```python
from build123d import *

# Parameters (mm, degrees)
F1_DEPTH = 161
F3_DEPTH = 161
F5_DEPTH = 161


with BuildPart() as f1:
    # F0 (on Top) → F1 (new body)
    with BuildSketch(Plane.XY):
        Polygon((800, 0), (0, 0), (0, -250), (28.50642, -318.820585), (81.179415, -371.49358), (150, -400), (800, -400), align=None)
    extrude(amount=-F1_DEPTH)

    # F2 (on face) → F3 (join)
    with BuildSketch(Plane(origin=(0, 0, -161), x_dir=(1, 0, 0), z_dir=(0, 0, -1))):
        Polygon((-191.910937, 466.098754), (-260, 301.717216), (-260, 0), (800, 0), (800, 660), (98.282784, 660), (-66.098754, 591.910937), align=None)
    extrude(amount=F3_DEPTH)

    # F4 (on face) → F5 (join)
    with BuildSketch(Plane(origin=(0, 0, -322), x_dir=(1, 0, 0), z_dir=(0, 0, -1))):
        Polygon((-412.328294, 613.376924), (-520, 353.434431), (-520, 0), (800, 0), (800, 920), (46.565569, 920), (-213.376924, 812.328294), align=None)
    extrude(amount=F5_DEPTH)


solid = f1.part
```
The model under review builds one solid part; all positions refer to its coordinate system, in mm. A direction names the side the tool comes from. Coordinates: 2 decimals unless noted, no trailing zeros. Order: outer loops, then holes, each group sorted by start corner. A loop starts at its lowest first (then second) coordinate and runs counter-clockwise, first axis right, second up. Notation, with made-up numbers: (42.5, 0.5) -> (91.5, 0.5) arc R23 cw to (91.5, 15.5) -> close; hole circle Ø2 at (84.25, -39.5). An arc over 180 degrees is marked (long way). Answer in a Markdown table with one row per item. Add a question column.
Item 1: We need section B-B on x = 546. Write out the cut boundary in (y, z).
Item 2: We need section C-C on z = -410. Write out the cut boundary in (x, y), plus the area to 3 significant figures.
Item 3: We need section D-D on z = -296. Write out the cut boundary in (x, y).
Item 4: We need section A-A on y = -159. Write out the cut boundary in (x, z).
Item 5: To check wall thickness, follow probe 1 along Z at (x, y) = (-190, -515); probe 2 along Z at (x, y) = (637, -542); probe 3 along X at (y, z) = (-105, -279). State the ranges of each line that lie inside material, in increasing order.
Item 6: Machinability: for faces 1 (the flat face through (454, -660, -240)), 2 (the flat face through (115.11, -385.55, -79.37)), 3 (the flat face through (-81.586, -866.918, -401.373)), 4 (the flat face through (-260, -153, -240)), which of the approach directions +Z, -Z, +X, -X, +Y, -Y give a long, thin tool a straight path to every point of the face, cutting with its end or side? Answer none if there is none.
Item 7: Clearance check with flat-ended pins moving along their axes: pin 1 (2 mm diameter, centred on x = 505.5, y = -748.5, fed in from +Z); pin 2 (2 mm diameter, centred on y = -513.5, z = -306, fed in from -X). State where each tip first meets the part, or that it passes through.
Final values:
| question | item | result |
|---|---|---|
| 1 | outline | (-920, -483) -> (0, -483) -> (0, 0) -> (-400, 0) -> (-400, -161) -> (-660, -161) -> (-660, -322) -> (-920, -322) -> close |
| 2 | outline | (-520, -353.43) -> (-412.33, -613.38) -> (-213.38, -812.33) -> (46.57, -920) -> (800, -920) -> (800, 0) -> (-520, 0) -> close |
| 2 | area | 1,110,000 mm2 |
| 3 | outline | (-260, -301.72) -> (-191.91, -466.1) -> (-66.1, -591.91) -> (98.28, -660) -> (800, -660) -> (800, 0) -> (-260, 0) -> close |
| 4 | outline | (-520, -483) -> (800, -483) -> (800, 0) -> (0, 0) -> (0, -161) -> (-260, -161) -> (-260, -322) -> (-520, -322) -> close |
| 5 | probe 1 | z = -483 to -322 |
| 5 | probe 2 | z = -483 to -161 |
| 5 | probe 3 | x = -260 to 800 |
| 6 | face 1 | +Z, +X, -X, -Y |
| 6 | face 2 | +Z, -X, -Y |
| 6 | face 3 | +Z, -Z, -X, -Y |
| 6 | face 4 | +Z, -X, +Y, -Y |
| 7 | pin 1 | stops at z = -322 |
| 7 | pin 2 | stops at x = -145.51 |
